```python
from build123d import *

# Parameters (mm, degrees)
CROQUIS1_R              = 1.7
SALIENTE_EXTRUIR1_DEPTH = 3.75
SALIENTE_EXTRUIR2_START = 0.63
CROQUIS2_R              = 3.15
SALIENTE_EXTRUIR2_DEPTH = 0.63
CROQUIS4_R              = 2.5
CORTAR_EXTRUIR1_DEPTH   = 1.8
SALIENTE_EXTRUIR3_START = 2.2
SALIENTE_EXTRUIR3_DEPTH = 2.2
CROQUIS6_R              = 2.3625
SALIENTE_EXTRUIR4_DEPTH = 28.6
SALIENTE_EXTRUIR5_START = 2.2
CROQUIS7_R              = 0.95
SALIENTE_EXTRUIR5_DEPTH = 2.2
CROQUIS8_R              = 1.25
CORTAR_EXTRUIR2_DEPTH   = 0.5


with BuildPart() as part:
    # Croquis1 → Saliente-Extruir1 (new body)
    with BuildSketch(Plane.XY):
        with BuildLine():
            Line((0, 3.15), (47.88, 3.15))
            ThreePointArc((47.88, 3.15), (51.03, 0), (47.88, -3.15))
            Line((47.88, -3.15), (0, -3.15))
            ThreePointArc((0, -3.15), (-3.15, 0), (0, 3.15))
        make_face()
        Circle(CROQUIS1_R, mode=Mode.SUBTRACT)
    extrude(amount=SALIENTE_EXTRUIR1_DEPTH)

    # Croquis2 → Saliente-Extruir2 (add)
    with BuildSketch(Plane(origin=(0, 0, 0), x_dir=(-1, 0, 0), z_dir=(0, 0, -1)).offset(SALIENTE_EXTRUIR2_START)):
        with Locations((-47.88, 0)):
            Circle(CROQUIS2_R)
    extrude(amount=-SALIENTE_EXTRUIR2_DEPTH)

    # Croquis4 → Cortar-Extruir1 (cut)
    with BuildSketch(Plane.XY.offset(3.75)):
        Circle(CROQUIS4_R)
    extrude(amount=-CORTAR_EXTRUIR1_DEPTH, mode=Mode.SUBTRACT)

    # Croquis5 → Saliente-Extruir3 (add)
    with BuildSketch(Plane(origin=(0, 0, -0.63), x_dir=(-1, 0, 0), z_dir=(0, 0, -1)).offset(SALIENTE_EXTRUIR3_START)):
        with BuildLine():
            Line((-51.03, 15.75), (-51.03, 0))
            ThreePointArc((-51.03, 0), (-47.88, -3.15), (-44.73, 0))
            Line((-44.73, 0), (-44.73, 15.75))
            ThreePointArc((-44.73, 15.75), (-47.88, 18.9), (-51.03, 15.75))
        make_face()
    extrude(amount=-SALIENTE_EXTRUIR3_DEPTH)

    # Croquis6 → Saliente-Extruir4 (add)
    with BuildSketch(Plane(origin=(0, 0, -2.83), x_dir=(-1, 0, 0), z_dir=(0, 0, -1))):
        with Locations((-47.88, 15.75)):
            Circle(CROQUIS6_R)
    extrude(amount=SALIENTE_EXTRUIR4_DEPTH)

    # Croquis7 → Saliente-Extruir5 (add)
    with BuildSketch(Plane(origin=(0, 0, -31.43), x_dir=(-1, 0, 0), z_dir=(0, 0, -1)).offset(SALIENTE_EXTRUIR5_START)):
        with BuildLine():
            Line((-51.03, 15.75), (-51.03, 0))
            ThreePointArc((-51.03, 0), (-47.88, -3.15), (-44.73, 0))
            Line((-44.73, 0), (-44.73, 15.75))
            ThreePointArc((-44.73, 15.75), (-47.88, 18.9), (-51.03, 15.75))
        make_face()
        with Locations((-47.88, 0)):
            Circle(CROQUIS7_R, mode=Mode.SUBTRACT)
    extrude(amount=-SALIENTE_EXTRUIR5_DEPTH)

    # Croquis8 → Cortar-Extruir2 (cut)
    with BuildSketch(Plane.XY.offset(-31.43)):
        with Locations((47.88, 0)):
            Circle(CROQUIS8_R)
    extrude(amount=-CORTAR_EXTRUIR2_DEPTH, mode=Mode.SUBTRACT)


solid = part.part
```
Geometry check sheet. Reference: the model listing, model coordinates, mm. A direction names the side the tool comes from. Give positions to 0.01 mm unless a question says otherwise; leave off trailing zeros. Order: outer loops, then holes, each group sorted by start corner. A loop starts at its lowest first (then second) coordinate and runs counter-clockwise, first axis right, second up.
1. Access from +Z, -Z, +X, -X, +Y, -Y to the whole of each face (thin tool, end or side, straight path). Record for faces 4 (the face through (44.73, 8, -2)), 5 (the face through (-0.54, -2.44, 2.86)), 6 (the face through (48.83, 0.04, -32.79)), 7 (the face through (47.95, -3.15, -32.55)), 8 (the face through (49.07, 0.38, -31.68)).
2. Section check A-A, the plane y = 6. Enter the section's corners in (x, z), and give its area (3 significant figures).
3. Section check C-C, the plane x = 10.5. Enter the section's corners in (y, z), and give its area (3 significant figures).
4. Gauge pin test, flat ends, axial feed: pin 1 Ø2.5 at (x, y) = (-1, 0) entering from +Z; pin 2 Ø1.5 at (x, y) = (47.88, 0) entering from -Z; pin 3 Ø2.5 at (y, z) = (8.5, -32.5) entering from -X. Record the tip position at first contact, or that the pin passes through.
5. Section check D-D, the plane y = 17. Enter the section's corners in (x, z).
6. Release check for a two-part mould opening along Z. For faces 1 (the face through (48.392, 13.444, -16.93)), 2 (the face through (51.03, 8, -33)), 3 (the face through (48, 8, -33.63)) record: pulls with the +Z half, pulls with the -Z half, needs draft (parallel to the pull), parting line crosses it, or undercut.
7. Thickness scan on L1, parallel to X at y = 0, z = 0.7; L2, parallel to Y at x = 47.88, z = -32.7; L3, parallel to Y at x = 24.5, z = 1.5. Record the ranges inside material, lowest first.
Values follow:
1. face 4: -Z, -X, +Y, -Y
1. face 5: +Z
1. face 6: -Z
1. face 7: -Z, -Y
1. face 8: none
2. outline: (44.73, -33.63) - (51.03, -33.63) - (51.03, -31.43) - (44.73, -31.43) - close; (44.73, -2.83) - (51.03, -2.83) - (51.03, -0.63) - (44.73, -0.63) - close
2. area: 27.7 mm2
3. outline: (-3.15, 0) - (3.15, 0) - (3.15, 3.75) - (-3.15, 3.75) - close
3. area: 23.6 mm2
4. pin 1: stops at z = 1.95
4. pin 2: stops at z = -2.83
4. pin 3: stops at x = 44.73
5. outline: (44.99, -33.63) - (50.77, -33.63) - (50.77, -31.43) - (49.88, -31.43) - (49.88, -2.83) - (50.77, -2.83) - (50.77, -0.63) - (44.99, -0.63) - (44.99, -2.83) - (45.88, -2.83) - (45.88, -31.43) - (44.99, -31.43) - close
6. face 1: undercut
6. face 2: needs draft
6. face 3: pulls with the -Z half
7. L1: x = -3.15 to -1.7, 1.7 to 51.03
7. L2: y = -3.15 to -0.95, 0.95 to 18.9
7. L3: y = -3.15 to 3.15
